```python
from build123d import *

# Parameters (mm, degrees)
SKETCH1_R           = 3
BOSS_EXTRUDE1_DEPTH = 9.38
BOSS_EXTRUDE2_DEPTH = 1
SKETCH5_R           = 2
BOSS_EXTRUDE3_DEPTH = 4
BOSS_EXTRUDE4_DEPTH = 1
CUT_EXTRUDE1_DEPTH  = 15
SKETCH8_W           = 1.762177923
SKETCH8_H           = 2.08
CUT_EXTRUDE2_DEPTH  = 5
CUT_REVOLVE2_ANGLE  = 180


with BuildPart() as part:
    # Sketch1 → Boss-Extrude1 (new body)
    with BuildSketch(Plane(origin=(0, 0, 0), x_dir=(1, 0, 0), z_dir=(0, 1, 0))):
        with BuildLine():
            Line((3, -8), (3, -19.1))
            ThreePointArc((3, -19.1), (3.263603897, -19.736396103), (3.9, -20))
            Line((3.9, -20), (4.1, -20))
            ThreePointArc((4.1, -20), (4.736396103, -19.736396103), (5, -19.1))
            Line((5, -19.1), (5, -8.5))
            ThreePointArc((5, -8.5), (5.878679656, -6.378679656), (8, -5.5))
            Line((8, -5.5), (10, -5.5))
            ThreePointArc((10, -5.5), (15.253803384, -3.323803384), (17.43, 1.93))
            Line((17.43, 1.93), (17.43, 3.3))
            Line((17.43, 3.3), (27.54785059, 3.3))
            Line((27.54785059, 3.3), (17.097491745, 8.1))
            Line((17.097491745, 8.1), (11.03, 4.5))
            Line((11.03, 4.5), (15.43, 4.5))
            Line((15.43, 4.5), (15.43, 1.93))
            ThreePointArc((15.43, 1.93), (13.839589822, -1.909589822), (10, -3.5))
            Line((10, -3.5), (8, -3.5))
            ThreePointArc((8, -3.5), (5.878679656, -2.621320344), (5, -0.5))
            Line((5, -0.5), (5, 0))
            ThreePointArc((5, 0), (-3.535533906, 3.535533906), (0, -5))
            ThreePointArc((0, -5), (2.121320344, -5.878679656), (3, -8))
        make_face()
        Circle(SKETCH1_R, mode=Mode.SUBTRACT)
    extrude(amount=BOSS_EXTRUDE1_DEPTH)

    # Sketch3 → Boss-Extrude2 (add, symmetric)
    with BuildSketch(Plane(origin=(0, 4.69, 0), x_dir=(1, 0, 0), z_dir=(0, 1, 0))):
        with BuildLine():
            Line((9.443635769, 1.375812361), (5.601654611, 1.375812361))
            ThreePointArc((5.601654611, 1.375812361), (4.981779837, 1.558852726), (4.560762938, 2.04925387))
            ThreePointArc((4.560762938, 2.04925387), (4.888957695, 1.047899163), (5, 0))
            Line((5, 0), (5, -0.5))
            ThreePointArc((5, -0.5), (5.878679656, -2.621320344), (8, -3.5))
            Line((8, -3.5), (10, -3.5))
            ThreePointArc((10, -3.5), (13.839589822, -1.909589822), (15.43, 1.93))
            Line((15.43, 1.93), (15.43, 4.5))
            Line((15.43, 4.5), (12.309861007, 4.5))
            Line((12.309861007, 4.5), (12.309861007, 4.242037598))
            ThreePointArc((12.309861007, 4.242037598), (11.470363071, 2.215310296), (9.443635769, 1.375812361))
        make_face()
    extrude(amount=BOSS_EXTRUDE2_DEPTH, both=True)

    # Sketch5 → Boss-Extrude3 (add)
    with BuildSketch(Plane.ZY.offset(-3)):
        with Locations((12.55, 4.69)):
            Circle(SKETCH5_R)
    extrude(amount=BOSS_EXTRUDE3_DEPTH)

    # Sketch6 → Boss-Extrude4 (add, symmetric)
    with BuildSketch(Plane(origin=(0, 4.69, 0), x_dir=(1, 0, 0), z_dir=(0, 1, 0))):
        with BuildLine():
            ThreePointArc((5, -8.5), (5.228361402, -7.351949703), (5.878679656, -6.378679656))
            Line((5.878679656, -6.378679656), (5.878679656, -18.972831199))
            Line((5.878679656, -18.972831199), (5, -18.972831199))
            Line((5, -18.972831199), (5, -8.5))
        make_face()
    extrude(amount=BOSS_EXTRUDE4_DEPTH, both=True)

    # Sketch7 → Cut-Extrude1 (cut)
    with BuildSketch(Plane(origin=(14, 0, 0), x_dir=(0, 0, -1), z_dir=(1, 0, 0))):
        with BuildLine():
            Line((-4.338573914, 9.38), (3.3, 22.365916212))
            Line((3.3, 22.365916212), (8.1, 10.195783218))
            Line((8.1, 10.195783218), (8.1, 7.3))
            Line((8.1, 7.3), (3.3, 7.3))
            ThreePointArc((3.3, 7.3), (-0.658352291, 7.829297677), (-4.338573914, 9.38))
        make_face()
    extrude(amount=CUT_EXTRUDE1_DEPTH, mode=Mode.SUBTRACT)

    # Sketch8 → Cut-Extrude2 (cut)
    with BuildSketch(Plane(origin=(14, 0, 0), x_dir=(0, 0, -1), z_dir=(1, 0, 0))):
        with Locations((5.381088961, 8.34)):
            Rectangle(SKETCH8_W, SKETCH8_H)
    extrude(amount=-CUT_EXTRUDE2_DEPTH, mode=Mode.SUBTRACT)

    # Sketch12 → Cut-Revolve2 (revolve, cut)
    with BuildSketch(Plane(origin=(14, 0, 0), x_dir=(0, 0, -1), z_dir=(1, 0, 0))):
        with BuildLine():
            Line((-1.74217919, 9.38), (-1.74217919, 8.168794661))
            ThreePointArc((-1.74217919, 8.168794661), (-3.065452427, 8.710776275), (-4.331381637, 9.375772039))
            Line((-4.331381637, 9.375772039), (-4.331381637, 10.213200203))
            Line((-4.331381637, 10.213200203), (-1.74217919, 10.213200203))
            Line((-1.74217919, 10.213200203), (-1.74217919, 9.38))
        make_face()
    revolve(axis=Axis((14, 22.365916212, -3.3), (0, -1, 0)), revolution_arc=CUT_REVOLVE2_ANGLE, mode=Mode.SUBTRACT)


solid = part.part
```
Can you work these out from the model? Positions are in its coordinate system, mm. A direction names the side the tool comes from. Give positions to 0.01 mm unless a question says otherwise; leave off trailing zeros. Order: outer loops, then holes, each group sorted by start corner. A loop starts at its lowest first (then second) coordinate and runs counter-clockwise, first axis right, second up. Notation, with made-up numbers: (13, 36.25) - (67, 36.25) arc R12 ccw to (67, 47.25) - close; hole circle Ø1 at (87.5, 58.25). An arc over 180 degrees is marked (long way). Use a Markdown table: item, result. Add a question column.
Q1. I'm going to push flat-ended pins straight in: pin 1 (2 mm diameter, centred on x = 8.5, y = 8, fed in from -Z); pin 2 (1 mm diameter, centred on x = 5, y = 8, fed in from +Z); pin 3 (1.3 mm diameter, centred on y = 2.5, z = -3, fed in from -X); pin 4 (8 mm diameter, centred on x = 15, z = 6.5, fed in from -Y). Where does each tip first touch, or does it pass through?
Q2. If we section it at A-A on y = 2: Write out the boundary of the cut face in (x, z), plus the area to 3 significant figures.
Q3. If we mould it in two halves opening along Z, with no side actions, what happens to faces 4 (the flat face through (22.396, 3.599, -5.666)), 5 (the flat face through (11, 5.69, 0)), 6 (the cylindrical face through (11.493, 4.704, -2.238)), 7 (the cylindrical face through (3.26, 4.62, 19.73))? For each: released by +Z, released by -Z, zero draft, split by the parting line, or undercut.
Q4. On a 3-axis mill with a long thin cutter (end or side, diameter ignored), from which of +Z, -Z, +X, -X, +Y, -Y can I reach the whole of each face in a straight line? I mean faces 1 (the cylindrical face through (15.691, 7.814, 0.6)), 2 (the flat face through (5.879, 5, 13)), 3 (the flat face through (15.43, 2, -3)). Say none if no direction works.
Q5. If we section it at B-B on z = -0.5: Write out the boundary of the cut face in (x, y), plus the area to 3 significant figures.
Q6. Please list where these lines run through material, in increasing order: line 1 along Z through (x, y) = (0, 2.5); line 2 along X through (y, z) = (6.25, 0); line 3 along X through (y, z) = (2.5, 1).
Q7. If we section it at C-C on x = 8.5: Write out the boundary of the cut face in (y, z).
Q8. If we section it at D-D on z = 12.55: Write out the boundary of the cut face in (x, y), plus the area to 3 significant figures.
Answers follow:
| question | item | result |
|---|---|---|
| 1 | pin 1 | stops at z = 3.46 |
| 1 | pin 2 | stops at z = 19.91 |
| 1 | pin 3 | stops at x = -4.41 |
| 1 | pin 4 | stops at y = 0 |
| 2 | outline | (0, 5) arc R5 ccw (long way) to (5, 0) - (5, 0.5) arc R3 cw to (8, 3.5) - (10, 3.5) arc R5.43 cw to (15.43, -1.93) - (15.43, -4.5) - (11.03, -4.5) - (17.1, -8.1) - (27.55, -3.3) - (17.43, -3.3) - (17.43, -1.93) arc R7.43 ccw to (10, 5.5) - (8, 5.5) arc R3 cw to (5, 8.5) - (5, 19.1) arc R0.9 ccw to (4.1, 20) - (3.9, 20) arc R0.9 ccw to (3, 19.1) - (3, 8) arc R3 cw to start; hole circle Ø6 at (0, 0) |
| 2 | area | 162 mm^2 |
| 3 | face 4 | released by -Z |
| 3 | face 5 | undercut |
| 3 | face 6 | undercut |
| 3 | face 7 | released by +Z |
| 4 | face 1 | -Z, +X, +Y |
| 4 | face 2 | +Z, +X, +Y, -Y |
| 4 | face 3 | -Y |
| 5 | outline | (-4.97, 0) - (-2.96, 0) - (-2.96, 9.38) - (-4.97, 9.38) - close; (2.96, 0) - (4.97, 0) - (4.97, 3.69) - (15.24, 3.69) - (15.24, 0) - (17.29, 0) - (17.29, 7.56) - (15.24, 7.56) - (15.24, 5.69) - (4.97, 5.69) - (4.97, 9.38) - (2.96, 9.38) - close |
| 5 | area | 73.9 mm^2 |
| 6 | line 1 | z = -5 to -3, 3 to 5 |
| 6 | line 2 | x = -5 to -3, 3 to 5, 15.08 to 17.17 |
| 6 | line 3 | x = -4.9 to -2.83, 2.83 to 5.04, 14.57 to 16.83 |
| 7 | outline | (0, 3.5) - (3.69, 3.5) - (3.69, -1.38) - (5.69, -1.38) - (5.69, 3.5) - (9.38, 3.5) - (9.38, 5.5) - (0, 5.5) - close |
| 8 | outline | (-1, 2.69) - (3, 2.69) - (3, 0) - (5, 0) - (5, 3.69) - (5.88, 3.69) - (5.88, 5.69) - (5, 5.69) - (5, 9.38) - (3, 9.38) - (3, 6.69) - (-1, 6.69) - close |
| 8 | area | 36.5 mm^2 |
